Geometry: final body of the model. Coordinates: model frame, mm. A direction names the side the tool comes from. Round coordinates to 2 decimals unless told otherwise and drop trailing zeros. Loops run counter-clockwise (first coordinate to the right, second up) from the corner with the lowest first, then second, coordinate; pieces in that order, holes last. Notation, with made-up numbers: M 61,87.5 L 86,87.5 A31 cw 86,113.5 Z; hole C 13.5,-5 d4. An arc over 180 degrees is marked long. Write each question's results on one line, items separated by ' | '.
```python
from build123d import *

# Parameters (mm, degrees)
SKETCH_1_R      = 9.5
EXTRUDE_1_DEPTH = 15
EXTRUDE_2_DEPTH = 1.5
SKETCH_4_R      = 8
EXTRUDE_3_DEPTH = 18


with BuildPart() as part:
    # 草图1 → 凸台-拉伸1 (new body)
    with BuildSketch(Plane.XY):
        Circle(SKETCH_1_R)
    extrude(amount=EXTRUDE_1_DEPTH)

    # 草图2 → 凸台-拉伸2 (add)
    with BuildSketch(Plane(origin=(0, 0, 0), x_dir=(-1, 0, 0), z_dir=(0, 0, -1))):
        Polygon((6.350852961, 11), (-6.350852961, 11), (-12.701705922, 0), (-6.350852961, -11), (6.350852961, -11), (12.701705922, 0), align=None)
    extrude(amount=-EXTRUDE_2_DEPTH)

    # 草图3 → 旋转1 (revolve)
    with BuildSketch(Plane(origin=(0, 0, 0), x_dir=(1, 0, 0), z_dir=(0, 1, 0))):
        with BuildLine():
            Line((0, 0), (0, 1.5))
            Line((0, 1.5), (-8.5, 1.5))
            ThreePointArc((-8.5, 1.5), (-9.924633098, 1.041055163), (-11, 0))
            Line((-11, 0), (0, 0))
        make_face()
    revolve(axis=Axis((0, 0, 0), (0, 0, -1)))

    # 草图4 → 凸台-拉伸3 (add)
    with BuildSketch(Plane.XY.offset(15)):
        Circle(SKETCH_4_R)
    extrude(amount=EXTRUDE_3_DEPTH)


solid = part.part
```
1. Section A-A (z = 29). Output: boundary loops of the cut face in (x, y).
Answer key:
outline: C 0,0 d16
2. Ray query, probe 1 along Y at (x, z) = (4.25, 4); probe 2 along X at (y, z) = (-7.75, 4); probe 3 along Z at (x, y) = (-8.25, 2). Return the intervals inside material, ascending.
Answer key:
probe 1: y = -8.5 to 8.5 | probe 2: x = -5.49 to 5.49 | probe 3: z = -1.5 to 15
3. Pin query (flat end, axial travel): P1, Ø3, axis at y = -5.5, z = 17.5, coming from the -X side; P2, Ø5, axis at x = 2.5, z = 12.5, coming from the +Y side; P3, Ø5, axis at x = -4.5, z = 16.5, coming from the +Y side. Return the tip coordinate at first contact, or that it passes through.
Answer key:
P1: stops at x = -6.93 | P2: stops at y = 9.5 | P3: stops at y = 9.17
4. Access query for faces 1 (the face through (-6, 10, 0)), 2 (the face through (-6, -10, 0)), 3 (the face through (-8.4, -4.8, 1.5)). Directions: +Z, -Z, +X, -X, +Y, -Y. A direction counts if a zero-diameter tool reaches every point of the face in a straight line with its end or side. Return the directions, or none.
Answer key:
face 1: -Z, -X, +Y | face 2: -Z, -X, -Y | face 3: +Z
